Geometry: final body of the model. Coordinates: model frame, mm. A direction names the side the tool comes from. Give positions to 0.01 mm unless a question says otherwise; leave off trailing zeros. Write each loop counter-clockwise with the first axis right and the second up, starting at its lowest first coordinate (ties: lowest second). Pieces come first, ordered by that corner, then holes. Notation, with made-up numbers: (20.25, -9.5) - (67.25, -9.5) arc R27 ccw to (67.25, 25.5) - close; hole circle Ø3 at (52, 36). An arc over 180 degrees is marked (long way). Return JSON: item names as keys, results as strings.
from build123d import *

# Parameters (mm, degrees)
SKETCH1_W           = 30
SKETCH1_H           = 50
BOSS_EXTRUDE1_DEPTH = 5
SKETCH5_R           = 3.175
CUT_EXTRUDE2_DEPTH  = 30.580398915
SKETCH2_W           = 5
SKETCH2_H           = 50
BOSS_EXTRUDE2_DEPTH = 2
SKETCH3_W           = 10
SKETCH3_H           = 50
BOSS_EXTRUDE3_DEPTH = 20
SKETCH4_R           = 3.5
CUT_EXTRUDE1_DEPTH  = 3
SKETCH6_R           = 9
CUT_EXTRUDE3_DEPTH  = 2
SKETCH7_W           = 32
SKETCH7_H           = 5
SKETCH7_W_2         = 20
SKETCH7_H_2         = 18
BOSS_EXTRUDE4_DEPTH = 5
FILLET1_R           = 10


with BuildPart() as part:
    # Sketch1 → Boss-Extrude1 (new body)
    with BuildSketch(Plane.XY):
        Rectangle(SKETCH1_W, SKETCH1_H)
    extrude(amount=BOSS_EXTRUDE1_DEPTH)

    # Sketch5 → Cut-Extrude2 (cut, through all)
    with BuildSketch(Plane.XY.offset(5)):
        with Locations((0, 12.5)):
            Circle(SKETCH5_R)
        with Locations((0, -12.5)):
            Circle(SKETCH5_R)
    extrude(amount=-CUT_EXTRUDE2_DEPTH, mode=Mode.SUBTRACT)

    # Sketch2 → Boss-Extrude2 (add)
    with BuildSketch(Plane(origin=(15, 0, 0), x_dir=(0, 0, -1), z_dir=(1, 0, 0))):
        with Locations((-2.5, 0)):
            Rectangle(SKETCH2_W, SKETCH2_H)
    extrude(amount=BOSS_EXTRUDE2_DEPTH)

    # Sketch3 → Boss-Extrude3 (add)
    with BuildSketch(Plane(origin=(17, 0, 0), x_dir=(0, 0, -1), z_dir=(1, 0, 0))):
        with Locations((-5, 0)):
            Rectangle(SKETCH3_W, SKETCH3_H)
    extrude(amount=BOSS_EXTRUDE3_DEPTH)

    # Sketch4 → Cut-Extrude1 (cut)
    with BuildSketch(Plane.XY.offset(10)):
        with Locations((27, 15)):
            Circle(SKETCH4_R)
        with Locations((27, -15)):
            Circle(SKETCH4_R)
    extrude(amount=-CUT_EXTRUDE1_DEPTH, mode=Mode.SUBTRACT)

    # Sketch6 → Cut-Extrude3 (cut)
    with BuildSketch(Plane(origin=(0, 0, 0), x_dir=(-1, 0, 0), z_dir=(0, 0, -1))):
        with Locations((0, 12.5)):
            Circle(SKETCH6_R)
        with Locations((0, -12.5)):
            Circle(SKETCH6_R)
    extrude(amount=-CUT_EXTRUDE3_DEPTH, mode=Mode.SUBTRACT)

    # Sketch7 → Boss-Extrude4 (add)
    with BuildSketch(Plane.XZ.offset(25)):
        with Locations((1, 2.5)):
            Rectangle(SKETCH7_W, SKETCH7_H)
        Polygon((17, 0), (37, 0), (37, 10), (17, 10), (17, 5), align=None)
        with Locations((27, 19)):
            Rectangle(SKETCH7_W_2, SKETCH7_H_2)
    extrude(amount=BOSS_EXTRUDE4_DEPTH)

    # Fillet1
    # the kernel refuses this fillet: 10 mm, written as the material it takes off along each edge
    with BuildSketch(Plane(origin=(17, 25, 5), x_dir=(0, -1, 0), z_dir=(0, 0, 1))) as fillet1_piece_1:
        with BuildLine():
            CenterArc((FILLET1_R, FILLET1_R), FILLET1_R, 180, 90)
            Line((0, FILLET1_R), (0, 0))
            Line((0, 0), (FILLET1_R, 0))
        make_face()
    extrude(amount=30, mode=Mode.SUBTRACT)
    with BuildSketch(Plane(origin=(37, 25, -25), x_dir=(0, -1, 0), z_dir=(0, 0, 1))) as fillet1_piece_2:
        with BuildLine():
            CenterArc((FILLET1_R, -FILLET1_R), FILLET1_R, 90, 90)
            Line((0, -FILLET1_R), (0, 0))
            Line((0, 0), (FILLET1_R, 0))
        make_face()
    extrude(amount=60, mode=Mode.SUBTRACT)
    with BuildSketch(Plane(origin=(37, 0, 28), x_dir=(0, 0, -1), z_dir=(0, -1, 0)), Plane(origin=(17, 0, 28), x_dir=(1, 0, 0), z_dir=(0, -1, 0))) as fillet1_piece_3:
        with BuildLine():
            CenterArc((FILLET1_R, -FILLET1_R), FILLET1_R, 90, 90)
            Line((0, -FILLET1_R), (0, 0))
            Line((0, 0), (FILLET1_R, 0))
        make_face()
    extrude(amount=55, mode=Mode.SUBTRACT)
    with BuildSketch(Plane(origin=(-15, -30, 30), x_dir=(0, 1, 0), z_dir=(0, 0, -1)), Plane(origin=(-15, 25, -25), x_dir=(0, -1, 0), z_dir=(0, 0, 1))) as fillet1_piece_4:
        with BuildLine():
            CenterArc((FILLET1_R, FILLET1_R), FILLET1_R, 180, 90)
            Line((0, FILLET1_R), (0, 0))
            Line((0, 0), (FILLET1_R, 0))
        make_face()
    extrude(amount=55, mode=Mode.SUBTRACT)


solid = part.part
Q1. Section query B-B, the plane y = -12.5. Return the cut outline in (x, z) (3 decimals), plus the area to 3 significant figures.
Answer key:
{"outline": "(-15, 0) - (-9, 0) - (-9, 2) - (-3.175, 2) - (-3.175, 5) - (-15, 5) - close; (3.175, 2) - (9, 2) - (9, 0) - (37, 0) - (37, 10) - (29.449, 10) - (29.449, 7) - (24.551, 7) - (24.551, 10) - (17, 10) - (17, 5) - (3.175, 5) - close", "area": "290 mm^2"}
Q2. Section query D-D, the plane y = 19.5. Return the cut outline in (x, z), plus the area to 3 significant figures.
Answer key:
{"outline": "(-13.93, 0) - (-5.66, 0) - (-5.66, 2) - (5.66, 2) - (5.66, 0) - (35.93, 0) - (35.93, 10) - (18.07, 10) - (18.07, 5) - (-13.93, 5) - close", "area": "316 mm^2"}
Q3. Mould query, pull axis Y, two halves, no side actions, for faces 1 (the cylindrical face through (30.233, 13.659, 8.521)), 2 (the flat face through (1, -2, 5)), 3 (the cylindrical face through (-11.99, -27.15, 2.54)), 4 (the flat face through (27, -25, 19)). Classes: pulls with the +Y half, pulls with the -Y half, needs draft (parallel to the pull), parting line crosses it, or undercut.
Answer key:
{"face 1": "undercut", "face 2": "needs draft", "face 3": "pulls with the -Y half", "face 4": "pulls with the +Y half"}
Q4. Section query C-C, the plane z = 8. Return the cut outline in (x, y), plus the area to 3 significant figures.
Answer key:
{"outline": "(17, -30) - (37, -30) - (37, 15) arc R10 ccw to (17, 15) - close; hole circle Ø7 at (27, -15); hole circle Ø7 at (27, 15)", "area": "980 mm^2"}
Q5. Material intervals for probe 1 along Y at (x, z) = (0, 3) (3 decimals); probe 2 along Y at (x, z) = (27, 8.95); probe 3 along Z at (x, y) = (10.5, 3), sorted ascending. Write a range as [from, to].
Answer key:
{"probe 1": "y = [-30, -15.675], [-9.325, 9.325], [15.675, 25]", "probe 2": "y = [-30, -18.5], [-11.5, 11.5], [18.5, 25]", "probe 3": "z = [0, 5]"}
Q6. Pin query (flat end, axial travel): P1, Ø9, axis at x = 3, y = 14, coming from the -Z side; P2, Ø9, axis at x = 27, y = -15, coming from the +Z side; P3, Ø21, axis at x = 4.5, y = 10, coming from the +Z side. Return the tip coordinate at first contact, or that it passes through.
Answer key:
{"P1": "stops at z = 2", "P2": "stops at z = 10", "P3": "stops at z = 5"}
Q7. Set-up query: faces 5 (the cylindrical face through (28.615, -18.105, 8.521)), 6 (the flat face through (17, -12, 9)), 7 (the cylindrical face through (30.63, 24.32, 6.04)), 8 (the flat face through (27, 0, 10)), 9 (the cylindrical face through (1.951, -21.286, 0.986)). Return all of +Z, -Z, +X, -X, +Y, -Y with unobstructed straight access to the full face (end or side cutting, diameter ignored); none if empty.
Answer key:
{"face 5": "+Z", "face 6": "+Z, -X, +Y, -Y", "face 7": "+Z, +Y", "face 8": "+Z, +X, -X, +Y", "face 9": "-Z"}
Q8. Section query A-A, the plane x = 0. Return the cut outline in (y, z) (3 decimals).
Answer key:
{"outline": "(-30, 0) - (-21.5, 0) - (-21.5, 2) - (-15.675, 2) - (-15.675, 5) - (-30, 5) - close; (-9.325, 2) - (-3.5, 2) - (-3.5, 0) - (3.5, 0) - (3.5, 2) - (9.325, 2) - (9.325, 5) - (-9.325, 5) - close; (15.675, 2) - (21.5, 2) - (21.5, 0) - (25, 0) - (25, 5) - (15.675, 5) - close"}
